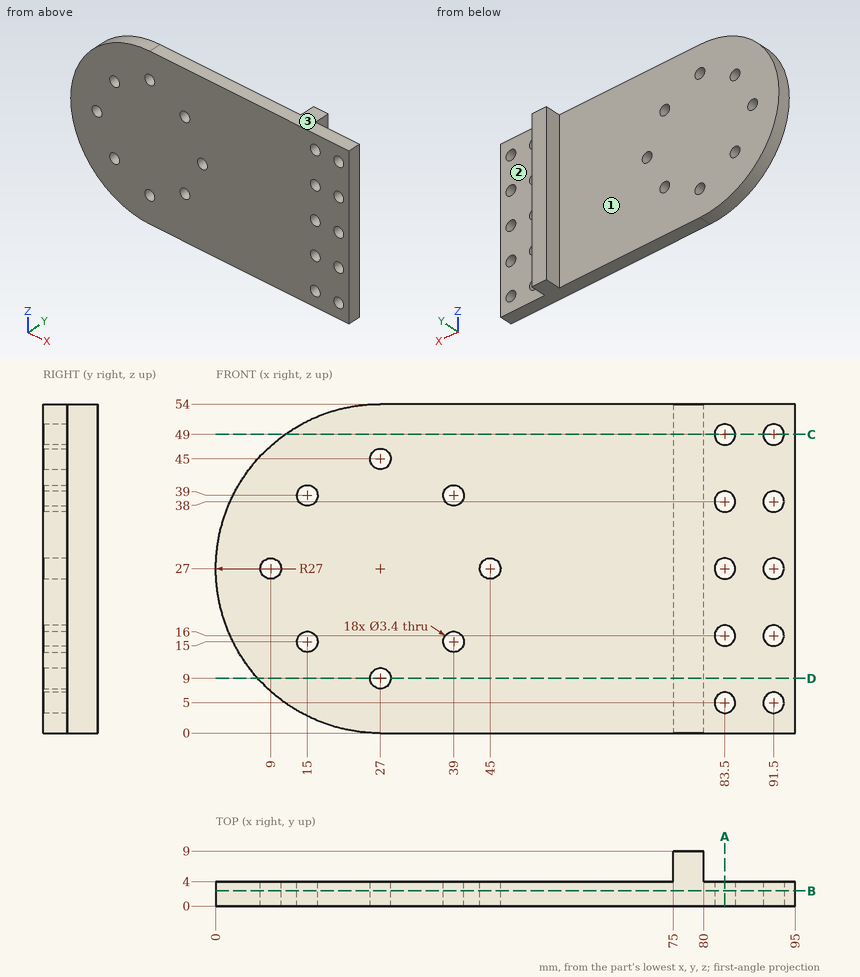
Geometry check sheet. Reference: drawing and pictorial views, mm from the part's lowest x, y, z. A direction names the side the tool comes from. Give positions to 0.01 mm unless a question says otherwise; leave off trailing zeros. Order: outer loops, then holes, each group sorted by start corner. A loop starts at its lowest first (then second) coordinate and runs counter-clockwise, first axis right, second up. Notation, with made-up numbers: M 2,2.5 L 11,2.5 A23 ccw 11,20.5 Z; hole C -30.5,5 d9. An arc over 180 degrees is marked long. Answer as a JSON object with one key per item and string values. Group by question number.
1) Scan lines: line 1 along Z through (x, y) = (91.5, 1.15); line 2 along Z through (x, y) = (27, 1.6); line 3 along Z through (x, y) = (39, 2.8). Record each from-to range of solid material in increasing order. Write a range as [from, to].
2) Cross-section at C-C (z = 49). Enter the section's corners in (x, y), then the cut area to 3 significant figures.
3) Cross-section at A-A (x = 83.5). Enter the section's corners in (y, z), then the cut area to 3 significant figures.
4) Depth check by flat-ended pin: pin 1 Ø3 at (x, z) = (15, 15) entering from -Y; pin 2 Ø5.5 at (x, z) = (83.5, 5) entering from +Y. Enter the tip coordinate at first touch or a pass-through.
5) Access from +Z, -Z, +X, -X, +Y, -Y to the whole of each face (thin tool, end or side, straight path). Record for the marked faces 1, 2 and 3.
6) Cross-section at B-B (y = 2.5). Give the number of separate pieces and of enclosed holes in the cut face, then the cut area to 3 significant figures.
7) Cross-section at D-D (z = 9). Enter the section's corners in (x, y).
Result sheet:
{
 "1": {"line 1": "z = [0, 3.3], [6.7, 14.3], [17.7, 25.3], [28.7, 36.3], [39.7, 47.3], [50.7, 54]", "line 2": "z = [0, 7.3], [10.7, 43.3], [46.7, 54]", "line 3": "z = [0, 13.3], [16.7, 37.3], [40.7, 54]"},
 "2": {"outline": "M 11.35,0 L 81.8,0 L 81.8,4 L 80,4 L 80,9 L 75,9 L 75,4 L 11.35,4 Z; M 85.2,0 L 89.8,0 L 89.8,4 L 85.2,4 Z; M 93.2,0 L 95,0 L 95,4 L 93.2,4 Z", "area": "332 mm2"},
 "3": {"outline": "M 0,0 L 4,0 L 4,3.3 L 0,3.3 Z; M 0,6.7 L 4,6.7 L 4,14.3 L 0,14.3 Z; M 0,17.7 L 4,17.7 L 4,25.3 L 0,25.3 Z; M 0,28.7 L 4,28.7 L 4,36.3 L 0,36.3 Z; M 0,39.7 L 4,39.7 L 4,47.3 L 0,47.3 Z; M 0,50.7 L 4,50.7 L 4,54 L 0,54 Z", "area": "148 mm2"},
 "4": {"pin 1": "passes through", "pin 2": "stops at y = 4"},
 "5": {"face 1": "+Z, -Z, -X, +Y", "face 2": "+Z, -Z, +X, +Y", "face 3": "+Z, +X, -X, +Y, -Y"},
 "6": {"separate pieces": "1", "enclosed holes": "18", "area": "4,650 mm2"},
 "7": {"outline": "M 6.88,0 L 25.3,0 L 25.3,4 L 6.88,4 Z; M 28.7,0 L 95,0 L 95,4 L 80,4 L 80,9 L 75,9 L 75,4 L 28.7,4 Z"}
}
